Source: CAD feature listing. Evaluate the final solid. Frame: model axes, mm. Face numbers are marked on the shaded views. A direction names the side the tool comes from. Round coordinates to 2 decimals unless told otherwise and drop trailing zeros. Loops run counter-clockwise (first coordinate to the right, second up) from the corner with the lowest first, then second, coordinate; pieces in that order, holes last. Notation, with made-up numbers: (66, 46) - (80, 46) arc R37 cw to (80, 84) - close; hole circle Ø1 at (23.5, -9). An arc over 180 degrees is marked (long way). One line per question, with ' | ' between items. Start each with the question number.
1. Cut plane C-C (x = 0). Return loops of the section in (y, z) (3 decimals).
2. Mould query, pull axis X, two halves, no side actions, for the marked faces 3, 4 and 5. Classes: pulls with the +X half, pulls with the -X half, needs draft (parallel to the pull), parting line crosses it, or undercut.
3. Cut plane D-D (y = 0). Return loops of the section in (x, z) (3 decimals), then the cut area to 4 significant figures.
4. Pin query (flat end, axial travel): pin 1 (5.5 mm diameter, centred on x = 0, y = 0, fed in from -Z). Return the tip coordinate at first contact, or that it passes through.
5. Cut plane A-A (y = 3.75). Return loops of the section in (x, z) (3 decimals).
6. Access query for the marked faces 1 and 2. Directions: +Z, -Z, +X, -X, +Y, -Y. A direction counts if a zero-diameter tool reaches every point of the face in a straight line with its end or side. Return the directions, or none.
7. Ray query, line 1 (X direction, y = 0, z = 0.8) (3 decimals); line 2 (Y direction, x = 0, z = 0.6) (3 decimals); line 3 (X direction, y = 2.5, z = 0.6) (3 decimals). Return the intervals inside material, ascending.
8. Cut plane B-B (z = 0.35). Return loops of the section in (x, y) (3 decimals).
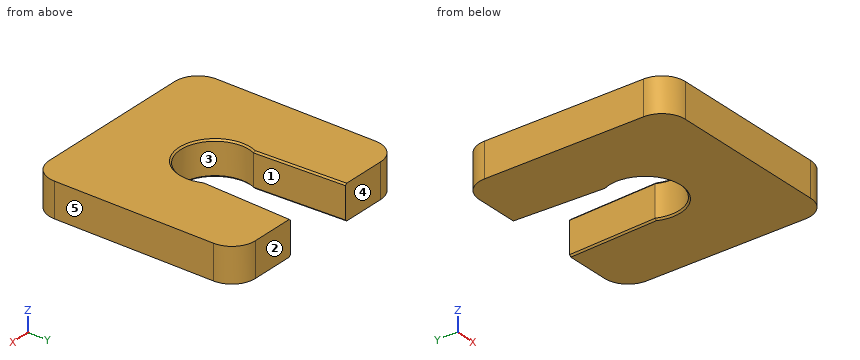
```python
from build123d import *

# Parameters (mm, degrees)
PAD_DEPTH       = 2.2
SKETCH001_R     = 2.2
POCKET_DEPTH    = 5
POCKET001_DEPTH = 5
CHAMFER_SIZE    = 0.1
CHAMFER001_SIZE = 0.1


with BuildPart() as part:
    # Sketch → Pad (new body)
    with BuildSketch(Plane.XY):
        with BuildLine():
            Line((-5.125, 6.625), (5.125, 6.625))
            ThreePointArc((6.625, 5.125), (6.18566, 6.18566), (5.125, 6.625))
            Line((6.625, 5.125), (6.625, -5.125))
            ThreePointArc((5.125, -6.625), (6.18566, -6.18566), (6.625, -5.125))
            Line((5.125, -6.625), (-5.125, -6.625))
            ThreePointArc((-6.625, -5.125), (-6.18566, -6.18566), (-5.125, -6.625))
            Line((-6.625, -5.125), (-6.625, 5.125))
            ThreePointArc((-5.125, 6.625), (-6.18566, 6.18566), (-6.625, 5.125))
        make_face()
    extrude(amount=PAD_DEPTH)

    # Sketch001 (on Face10 of Pad) → Pocket (cut)
    with BuildSketch(Plane.XY.offset(2.2)):
        Circle(SKETCH001_R)
    extrude(amount=-POCKET_DEPTH, mode=Mode.SUBTRACT)

    # Sketch002 (on Face5 of Pocket) → Pocket001 (cut)
    with BuildSketch(Plane.XY.offset(2.2)):
        with BuildLine():
            Line((-2, 0.902418), (-2.249768, 6.693066))
            ThreePointArc((-2, 6.95384), (-2.180545, 6.876765), (-2.249768, 6.693066))
            Line((-2, 6.95384), (2, 6.95384))
            ThreePointArc((2.249768, 6.693066), (2.180545, 6.876765), (2, 6.95384))
            Line((2.249768, 6.693066), (2, 0.902418))
            Line((2, 0.902418), (-2, 0.902418))
        make_face()
    extrude(amount=-POCKET001_DEPTH, mode=Mode.SUBTRACT)

    # Chamfer
    chamfer_edges = [part.edges().sort_by_distance(p)[0] for p in [
        (-2.123694, 3.770151, 2.2),
        (-0.46839, -2.149561, 2.2),
        (2.149561, 0.46839, 2.2),
        (2.123694, 3.770151, 2.2),
    ]]
    chamfer(chamfer_edges, length=CHAMFER_SIZE)

    # Chamfer001
    chamfer001_edges = [part.edges().sort_by_distance(p)[0] for p in [
        (2.149561, 0.46839, 0),
        (2.123694, 3.770151, 0),
        (-0.46839, -2.149561, 0),
        (-2.123694, 3.770151, 0),
    ]]
    chamfer(chamfer001_edges, length=CHAMFER001_SIZE)


solid = part.part
```
Answers follow:
1) outline: (-6.625, 0) - (-2.3, 0) - (-2.2, 0.1) - (-2.2, 2.1) - (-2.3, 2.2) - (-6.625, 2.2) - close
2) face 3: undercut | face 4: needs draft | face 5: pulls with the +X half
3) outline: (-6.625, 0) - (-2.3, 0) - (-2.2, 0.1) - (-2.2, 2.1) - (-2.3, 2.2) - (-6.625, 2.2) - close; (2.2, 0.1) - (2.3, 0) - (6.625, 0) - (6.625, 2.2) - (2.3, 2.2) - (2.2, 2.1) - close | area: 19.45 mm2
4) pin 1: stops at z = 0
5) outline: (-6.625, 0) - (-2.223, 0) - (-2.123, 0.1) - (-2.123, 2.1) - (-2.223, 2.2) - (-6.625, 2.2) - close; (2.123, 0.1) - (2.223, 0) - (6.625, 0) - (6.625, 2.2) - (2.223, 2.2) - (2.123, 2.1) - close
6) face 1: +Z, -Z, +Y | face 2: +Z, -Z, +X, -X, +Y
7) line 1: x = -6.625 to -2.2, 2.2 to 6.625 | line 2: y = -6.625 to -2.2 | line 3: x = -6.625 to -2.069, 2.069 to 6.625
8) outline: (-6.625, -5.125) arc R1.5 ccw to (-5.125, -6.625) - (5.125, -6.625) arc R1.5 ccw to (6.625, -5.125) - (6.625, 5.125) arc R1.5 ccw to (5.125, 6.625) - (2.247, 6.625) - (2.001, 0.915) arc R2.2 cw (long way) to (-2.001, 0.915) - (-2.247, 6.625) - (-5.125, 6.625) arc R1.5 ccw to (-6.625, 5.125) - close
